Verification items for the finished model (mm, model axes). A direction names the side the tool comes from. Coordinates: 2 decimals unless noted, no trailing zeros. Write each loop counter-clockwise with the first axis right and the second up, starting at its lowest first coordinate (ties: lowest second). Pieces come first, ordered by that corner, then holes. Notation, with made-up numbers: (89, -18.75) - (119, -18.75) arc R32 cw to (119, 20.25) - close; hole circle Ø6 at (-24, 24). An arc over 180 degrees is marked (long way). Use CSV: the item, a comma, the result in double quotes. Start each with the question number.
Autodesk Inventor part; units mm, degrees
ref_plane "YZ Plane" through (0, 0, 0) normal (1, 0, 0) x (0, 1, 0)
ref_plane "XZ Plane" through (0, 0, 0) normal (0, 1, 0) x (-1, 0, 0)
ref_plane "XY Plane" through (0, 0, 0) normal (0, 0, 1) x (1, 0, 0)
sketch "Эскиз1" plane through (0, 0, 0) normal (0, 1, 0) x (-1, 0, 0)
  circle A0 centre (0, 0) radius 5
  circle A1 centre (0, 0) radius 2.5
  circle A2 centre (0, 0) radius 11
  circle A3 centre (8, 0) radius 1.5
  circle A4 centre (-8, 0) radius 1.5
  circle A5 centre (0, 8) radius 1.5
  circle A6 centre (0, -8) radius 1.5
  dimension "d0" = 5
  dimension "d1" = 10
  dimension "d2" = 22
  dimension "d3" = 3
  dimension "d4" = 3
  dimension "d5" = 16
  dimension "d6" = 8
  dimension "d7" = 3
  dimension "d8" = 3
  dimension "d9" = 8
  dimension "d10" = 8
  dimension "d11" = 16
extrude "Выдавливание1" add sketch "Эскиз1" along normal blind 2 contours A2
extrude "Выдавливание2" add sketch "Эскиз1" along normal blind 10 contours A0
sketch "Эскиз2" plane through (0, 0, 0) normal (1, 0, 0) x (0, 1, 0)
  point P0 (0, 0)
  point P1 (-0.4556, -12.0524)
  point P2 (8.9773, -12.0404)
sketch "Эскиз3" plane through (0, 0, 0) normal (0, 0, 1) x (1, 0, 0)
  point P0 (0, 0)
  point P1 (-11.9191, -0.1213)
  point P2 (-11.9191, 9.5232)
ref_plane "РабПлоскость1" through (0, -0.4556, -12.0524) normal (0.711, -0.0009, 0.7032) x (0, 1, 0.0013)
sketch "Эскиз4" plane through (0, -0.4556, -12.0524) normal (0.711, -0.0009, 0.7032) x (0, 1, 0.0013)
  circle A0 centre (6.1565, 8.569) radius 1.5
  point P0 (0.4709, 8.569)
  dimension "d16" = 3
extrude "Выдавливание3" cut sketch "Эскиз4" along normal up to surface
properties part number "Муфта"
Q1. Cross-section at D-D (z = -8.75). Record the cut outline in (x, y).
Q2. Release check for a two-part mould opening along Y. For faces 1 (the cylindrical face through (-2.91, 7.074, -2.061)), 2 (the cylindrical face through (-6.5, 0.99, -0.07)), 3 (the flat face through (-2, 2, -5)) record: released by +Y, released by -Y, zero draft, split by the parting line, or undercut.
Q3. Scan lines: line 1 along Z through (x, y) = (0, 1.4); line 2 along Y through (x, z) = (5.5, 6.75); line 3 along X through (y, z) = (4.5, -0.5). Record each from-to range of solid material in increasing order. Write a range as from..to.
Q4. Gauge pin test, flat ends, axial feed: pin 1 (2.5 mm diameter, centred on x = 0, z = 8, fed in from -Y); pin 2 (1.5 mm diameter, centred on x = 0, y = 5.5, fed in from -Z); pin 3 (1.5 mm diameter, centred on y = 7, z = 2.5, fed in from -X); pin 4 (5 mm diameter, centred on y = 6, z = 0.5, fed in from +X). Record the tip position at first contact, or that the pin passes through.
Q5. Cross-section at A-A (z = 0). Record the cut outline in (x, y), plus the area to 3 significant figures.
Q6. Cross-section at B-B (x = 0). Record the cut outline in (y, z), plus the area to 3 significant figures.
Q7. Tool access check on faces 4 (the cylindrical face through (9.5, 0.99, -0.07)), 5 (the cylindrical face through (1.08, 5.94, 4.88)). Record the directions out of +Z, -Z, +X, -X, +Y, -Y that give a thin tool (end or side, any length) a straight path to the whole face; none if there is none.
Q8. Cross-section at C-C (y = 1.25). Record the cut outline in (x, z).
Reply:
1,outline,"(-6.67, 0) - (-1.3, 0) - (-1.3, 2) - (-6.67, 2) - close; (1.3, 0) - (6.67, 0) - (6.67, 2) - (1.3, 2) - close"
2,face 1,"undercut"
2,face 2,"zero draft"
2,face 3,"released by +Y"
3,line 1,"-11..-9.5, -6.5..-2.5, 2.5..6.5, 9.5..11"
3,line 2,"0..2"
3,line 3,"-4.97..-2.45, 2.45..4.97"
4,pin 1,"through"
4,pin 2,"z = -5"
4,pin 3,"x = -4.68"
4,pin 4,"x = 5"
5,outline,"(-11, 0) - (-9.5, 0) - (-9.5, 2) - (-11, 2) - close; (-6.5, 0) - (-2.5, 0) - (-2.5, 10) - (-5, 10) - (-5, 2) - (-6.5, 2) - close; (2.5, 0) - (6.5, 0) - (6.5, 2) - (5, 2) - (5, 10) - (2.5, 10) - close; (9.5, 0) - (11, 0) - (11, 2) - (9.5, 2) - close"
5,area,"62.0 mm^2"
6,outline,"(0, -11) - (2, -11) - (2, -9.5) - (0, -9.5) - close; (0, -6.5) - (2, -6.5) - (2, -5) - (10, -5) - (10, -2.5) - (0, -2.5) - close; (0, 2.5) - (10, 2.5) - (10, 5) - (2, 5) - (2, 6.5) - (0, 6.5) - close; (0, 9.5) - (2, 9.5) - (2, 11) - (0, 11) - close"
6,area,"62.0 mm^2"
7,face 4,"+Y, -Y"
7,face 5,"+Y"
8,outline,"circle Ø22 at (0, 0); hole circle Ø3 at (-8, 0); hole circle Ø5 at (0, 0); hole circle Ø3 at (0, -8); hole circle Ø3 at (0, 8); hole circle Ø3 at (8, 0)"
